Autodesk Inventor part; units mm, degrees
ref_plane "YZ Plane" through (0, 0, 0) normal (1, 0, 0) x (0, 1, 0)
ref_plane "XZ Plane" through (0, 0, 0) normal (0, 1, 0) x (-1, 0, 0)
ref_plane "XY Plane" through (0, 0, 0) normal (0, 0, 1) x (1, 0, 0)
sketch "Sketch1" plane through (0, 0, 0) normal (0, 0, 1) x (1, 0, 0)
  line L0 (0, 0) -> (25, 0)
  line L1 (25, 0) -> (25, 40)
  line L2 (25, 40) -> (0, 40)
  line L3 (0, 40) -> (0, 0)
  dimension "d1" = 25
  dimension "d2" = 40
  dimension "d3" = 25
extrude "Extrusion1" add sketch "Sketch1" against normal blind 30
sketch "Sketch2" plane through (25, 0, 0) normal (1, 0, 0) x (0, 0, -1)
  line L0 (0, 0) -> (30, 0)
  circle A0 centre (15, 6.56) radius 2.46
extrude "Extrusion2" cut sketch "Sketch2" against normal blind 30
sketch "Sketch3" plane through (0, 0, 0) normal (-1, 0, 0) x (0, 0, 1)
  line L0 (0, 0) -> (-30, 0)
  line L1 (-25.05, 0) -> (-4.95, 0)
  line L2 (-4.95, 0) -> (-4.95, 33.12)
  line L3 (-4.95, 33.12) -> (-25.05, 33.12)
  line L4 (-25.05, 33.12) -> (-25.05, 0)
  dimension "d11" = 20.1
extrude "Extrusion3" cut sketch "Sketch3" against normal blind 20
sketch "Sketch4" plane through (0, 0, 0) normal (0, -1, 0) x (1, 0, 0)
  line L0 (20, -4.95) -> (20, -25.05)
  line L1 (20, -15) -> (25, -15)
  line L2 (25, 0) -> (25, -30)
  line L3 (20, -8.025) -> (25, -8.025)
  line L4 (25, -8.025) -> (25, -21.975)
  line L5 (25, -21.975) -> (20, -21.975)
  line L6 (20, -21.975) -> (20, -8.025)
  line L7 (20, -8.025) -> (25, -21.975) construction
  line L8 (25, -8.025) -> (20, -21.975) construction
  line L9 (25, -12.54) -> (25, -17.46)
  point P0 (0, 0)
  point P1 (22.5, -15)
  dimension "d14" = 13.95
extrude "Extrusion4" add sketch "Sketch4" along normal blind 15
sketch "Sketch5" plane through (20, 0, 0) normal (-1, 0, 0) x (0, 0, 1)
  circle A0 centre (-15, 6.56) radius 2.46
  circle A1 centre (-15, 6.56) radius 4.7025
  circle A2 centre (-15, 6.56) radius 2.46
  circle A3 centre (-15, 6.56) radius 2.46
  point P0 (0, 0)
  dimension "d17" = 9.405
extrude "Extrusion5" cut sketch "Sketch5" against normal blind 2.1
sketch "Sketch6" plane through (25, 0, 0) normal (1, 0, 0) x (0, 0, -1)
  circle A0 centre (15, 6.56) radius 4.7025
  line L0 (15, 6.56) -> (15, 23.56)
  circle A1 centre (15, 23.56) radius 2.46
  point P0 (0, 0)
  dimension "d20" = 17
  dimension "d21" = 4.92
extrude "Extrusion6" cut sketch "Sketch6" against normal blind 10 contours A1
sketch "Sketch7" plane through (20, 0, 0) normal (-1, 0, 0) x (0, 0, 1)
  circle A0 centre (-15, 23.56) radius 2.46
  circle A1 centre (-15, 23.56) radius 4.7025
  point P0 (0, 0)
  dimension "d24" = 9.405
extrude "Extrusion7" cut sketch "Sketch7" against normal blind 2.1
sketch "Sketch9" plane through (25, 0, 0) normal (1, 0, 0) x (0, 0, -1)
  circle A0 centre (15, 6.56) radius 2.46
  circle A1 centre (15, 6.56) radius 2.46
  circle A2 centre (15, 23.56) radius 2.46
  circle A3 centre (15, 23.56) radius 2.46
  line L0 (30, 40) -> (30, 0)
  line L1 (30, 0) -> (30, 40)
  line L2 (30, 40) -> (0, 40)
  line L3 (0, 40) -> (0, 0)
  line L4 (0, 0) -> (8.025, 0)
  line L5 (21.975, 0) -> (21.975, -15)
  line L6 (21.975, -15) -> (8.025, -15)
  line L7 (8.025, -15) -> (8.025, 0)
  line L8 (0, 0) -> (8.025, 0)
  line L9 (21.975, 0) -> (30, 0)
extrude "Extrusion8" add sketch "Sketch9" along normal blind 5
sketch "Sketch10" plane through (0, 40, 0) normal (0, 1, 0) x (1, 0, 0)
  line L0 (0, 30) -> (30, 30)
  line L1 (30, 0) -> (0, 0)
  line L2 (0, 30) -> (30, 30)
  line L3 (30, 30) -> (30, 0)
  line L4 (30, 0) -> (0, 0)
  line L5 (0, 0) -> (0, 30)
extrude "Extrusion9" add sketch "Sketch10" along normal blind 30
sketch "Sketch12" plane through (30, 0, 0) normal (1, 0, 0) x (0, 0, -1)
  circle A0 centre (15, 6.56) radius 2.46
  line L0 (15, 6.56) -> (15, 15.06)
  circle A1 centre (15, 15.06) radius 2.525
  point P0 (0, 0)
  dimension "d31" = 8.5
  dimension "d33" = 5.05
extrude "Extrusion10" cut sketch "Sketch12" against normal blind 30 contours A1
sketch "Sketch14" plane through (0, 0, 0) normal (0, 0, 1) x (1, 0, 0)
  line L0 (30, 70) -> (0, 70)
  line L1 (0, 100) -> (-8, 100)
  line L2 (30, 0) -> (30, 70)
  line L3 (30, 118) -> (30, 70)
  line L4 (30, 105) -> (30, 100)
  line L5 (0, 70) -> (30, 70)
  line L6 (0, 70) -> (0, 100)
  line L7 (30, 122.5) -> (30, 118)
  line L8 (30, 70) -> (30, 145)
  line L9 (-2, 157.5) -> (-8, 160)
  line L10 (-2, 102.5) -> (-8, 100)
  line L11 (4, 130) -> (-2, 102.5)
  line L12 (4, 130) -> (-2, 157.5)
  line L13 (-8, 160) -> (15, 160)
  line L14 (30, 145) -> (15, 160)
  point P0 (0, 0)
  dimension "d47" = 30
extrude "Extrusion12" add sketch "Sketch14" against normal blind 30
sketch "Sketch15" plane through (0, 0, -25.05) normal (-1, 0, 0) x (0, 0, 1)
  line L0 (0, 33.12) -> (20.1, 33.12)
  line L1 (20.1, 33.12) -> (20.1, 0)
  line L2 (0, 33.12) -> (20.1, 33.12)
  line L3 (20.1, 33.12) -> (20.1, 31.1)
  line L4 (20.1, 31.1) -> (0, 31.1)
  line L5 (0, 31.1) -> (0, 33.12)
  point P0 (25.05, 0)
  dimension "d57" = 2.02
extrude "Extrusion13" add sketch "Sketch15" against normal blind 20
sketch "Sketch27" plane through (0, 0, 0) normal (0, 0, 1) x (1, 0, 0)
  point P0 (0, 0)
properties part number "55mm_x_30mm"
CAD build for the part. Positions are in the model's coordinates, mm. A direction names the side the tool comes from. Coordinates: 2 decimals unless noted, no trailing zeros. Order: outer loops, then holes, each group sorted by start corner. A loop starts at its lowest first (then second) coordinate and runs counter-clockwise, first axis right, second up.
Item 1: Band-saw the part on C-C on z = -15. Give the number of separate pieces and of enclosed holes in the cut face, plus the area to 3 significant figures.
Check sheet entries:
separate pieces: 4
enclosed holes: 0
area: 4,020 mm2
Item 2: Band-saw the part on B-B on y = 6.56. List the corners of the cut face in (x, z), plus the area to 3 significant figures.
Check sheet entries:
outline: (0, -30) - (30, -30) - (30, -17.46) - (22.1, -17.46) - (22.1, -19.7) - (20, -19.7) - (20, -25.05) - (0, -25.05) - close; (0, -4.95) - (20, -4.95) - (20, -10.3) - (22.1, -10.3) - (22.1, -12.54) - (30, -12.54) - (30, 0) - (0, 0) - close
area: 439 mm2
Item 3: Band-saw the part on A-A on x = 24.5. List the corners of the cut face in (y, z) (3 decimals).
Check sheet entries:
outline: (-15, -21.975) - (0, -21.975) - (0, -30) - (150.5, -30) - (150.5, 0) - (0, 0) - (0, -8.025) - (-15, -8.025) - close; hole circle Ø4.92 at (6.56, -15); hole circle Ø5.05 at (15.06, -15); hole circle Ø4.92 at (23.56, -15)
Item 4: Drill centre lines: L1, parallel to Z at x = 10.5, y = 18; L2, parallel to Y at x = 20.7, z = -15 (1 decimal); L3, parallel to Z at x = 28, y = 23.56. Where is each one in solid material? Low to high.
Check sheet entries:
L1: z = -30 to -25.05, -4.95 to 0
L2: y = -15 to 1.9, 11.3 to 12.5, 17.6 to 18.9, 28.3 to 154.3
L3: z = -30 to -17.46, -12.54 to 0
Item 5: Two-plate mould, pull along Y, no slides. Class faces 1 (the face through (10, 31.1, -15)), 2 (the face through (3, 160, -15)), 3 (the face through (25.07, 15.171, -12.477)), 4 (the face through (25.995, 7.502, -17.272)): +Y half, -Y half, draft (parallel to the pull), parting line (faces both ways), or undercut.
Check sheet entries:
face 1: -Y half
face 2: +Y half
face 3: undercut
face 4: undercut
Item 6: Band-saw the part on D-D on z = -23.5. List the corners of the cut face in (x, y).
Check sheet entries:
outline: (-8, 100) - (0, 100) - (0, 31.1) - (20, 31.1) - (20, 0) - (30, 0) - (30, 145) - (15, 160) - (-8, 160) - (-2, 157.5) - (4, 130) - (-2, 102.5) - close
Item 7: Pin check, flat tips, straight feed: pin 1 Ø10 at (y, z) = (36, -26) entering from -X; pin 2 Ø7.5 at (y, z) = (24, -17) entering from -X; pin 3 Ø9 at (x, z) = (13, -3) entering from -Y; pin 4 Ø4.5 at (y, z) = (6.56, -15) entering from +X. Stop position of each tip, or through.
Check sheet entries:
pin 1: stops at x = 0
pin 2: stops at x = 20
pin 3: stops at y = 0
pin 4: passes through
Item 8: 3-axis set-ups, long thin cutter, end or side, ignore diameter. For faces 5 (the face through (22.1, 21.5, -13)), 6 (the face through (-4, 100, -15)), 7 (the face through (20, 8, -20)), 8 (the face through (15, 0, -3)), 9 (the face through (25, -7, -21.975)): which of +Z, -Z, +X, -X, +Y, -Y reach the whole face in a straight line?
Check sheet entries:
face 5: -X
face 6: +Z, -Z, -X, -Y
face 7: -X, -Y
face 8: +Z, +X, -X, -Y
face 9: -Z, +X, -X, -Y
